Source: three-view drawing plus pictorial views. Frame: mm from the lowest corner of the part. Give positions to 0.01 mm unless a question says otherwise; leave off trailing zeros. Write each loop counter-clockwise with the first axis right and the second up, starting at its lowest first coordinate (ties: lowest second). Pieces come first, ordered by that corner, then holes.
Q1. Cut plane A-A on x = 40. Return the cut outline in (y, z), plus the area to 3 significant figures.
Q2. Draft query along X for the marked faces 1, 2 and 3. Return one class per face: pulls with the +X half, pulls with the -X half, needs draft (parallel to the pull), parting line crosses it, or undercut.
Q3. Pin query (flat end, axial travel): pin 1 (8 mm diameter, centred on y = 44, z = 68.5, fed in from -X). Return the tip coordinate at first contact, or that it passes through.
Q4. Line query: L1, parallel to Y at x = 40, z = 46; L2, parallel to X at y = 45.5, z = 61; L3, parallel to X at y = 32, z = 72.5. Output: solid intervals per line, ascending.
Q5. Cut plane C-C on z = 41.5. Return the cut outline in (x, y).
Q6. Cut plane B-B on y = 54. Return the cut outline in (x, z).
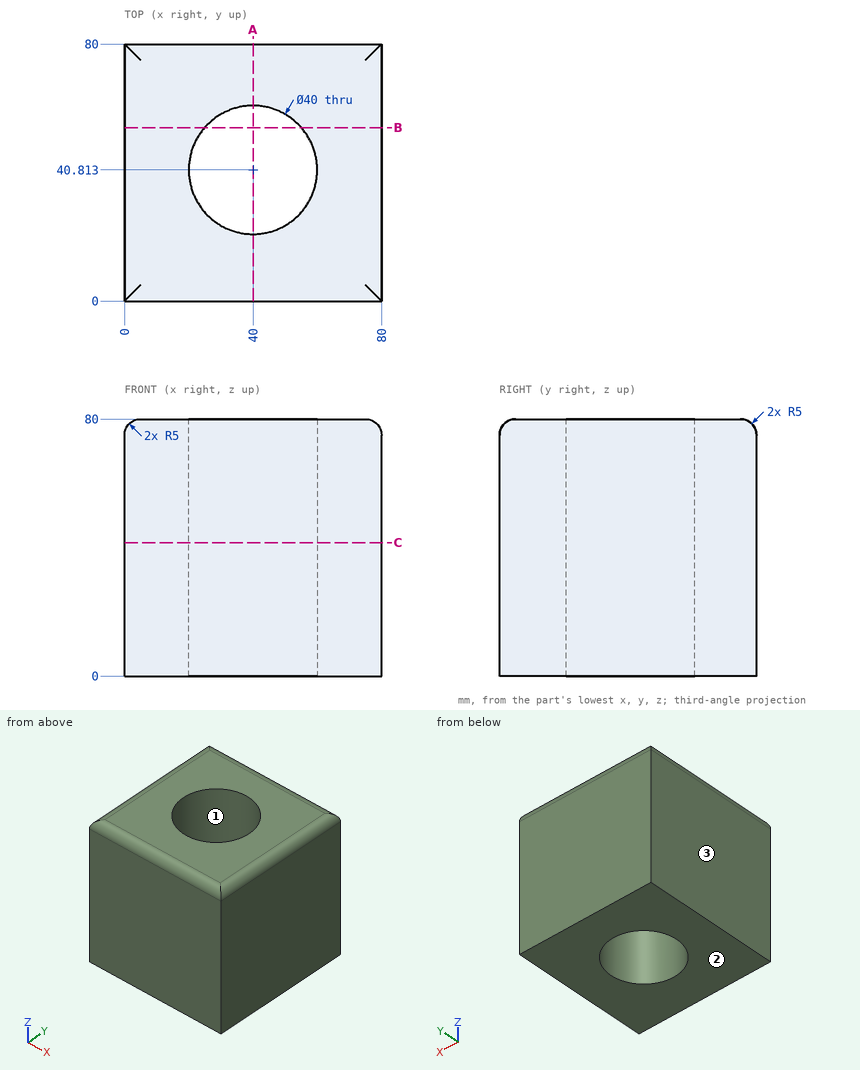
Data:
1. outline: (0, 0) - (20.81, 0) - (20.81, 80) - (5, 80) arc R5 ccw to (0, 75) - close; (60.81, 0) - (80, 0) - (80, 75) arc R5 ccw to (75, 80) - (60.81, 80) - close
1. area: 3,190 mm2
2. face 1: undercut
2. face 2: needs draft
2. face 3: pulls with the -X half
3. pin 1: stops at x = 0
4. L1: y = 0 to 20.81, 60.81 to 80
4. L2: x = 0 to 20.56, 59.44 to 80
4. L3: x = 0 to 22.05, 57.95 to 80
5. outline: (0, 0) - (80, 0) - (80, 80) - (0, 80) - close; hole circle Ø40 at (40, 40.81)
6. outline: (0, 0) - (24.96, 0) - (24.96, 80) - (5, 80) arc R5 ccw to (0, 75) - close; (55.04, 0) - (80, 0) - (80, 75) arc R5 ccw to (75, 80) - (55.04, 80) - close
